from build123d import *

# Parameters (mm, degrees)
BOSS_EXTRUDE1_DEPTH = 6.35


with BuildPart() as part:
    # Sketch1 → Boss-Extrude1 (new body)
    with BuildSketch(Plane(origin=(0, 0, 0), x_dir=(1, 0, 0), z_dir=(0, 1, 0))):
        with BuildLine():
            Line((1.248119104, -4.675816263), (2.497415053, -4.675816263))
            Line((2.497415053, -4.675816263), (2.497415053, -2.923216263))
            Line((2.497415053, -2.923216263), (5.037415053, -2.923216263))
            Line((5.037415053, -2.923216263), (5.037415053, -4.675816263))
            Line((5.037415053, -4.675816263), (8.212415053, -4.675816263))
            Line((8.212415053, -4.675816263), (8.212415053, -3.02471078))
            Line((8.212415053, -3.02471078), (8.212415053, 3.32528922))
            Line((8.212415053, 3.32528922), (14.562415053, 3.32528922))
            Line((14.562415053, 3.32528922), (14.562415053, 9.67528922))
            Line((14.562415053, 9.67528922), (8.212415053, 9.67528922))
            Line((8.212415053, 9.67528922), (-101.041741874, -93.72811078))
            ThreePointArc((-101.041741874, -93.72811078), (-118.331248541, -106.150388972), (-137.459794183, -115.49591078))
            Line((-137.459794183, -115.49591078), (-137.459794183, -123.496945941))
            Line((-137.459794183, -123.496945941), (-134.284794183, -123.496945941))
            Line((-134.284794183, -123.496945941), (-134.284794183, -121.744345941))
            Line((-134.284794183, -121.744345941), (-131.744794183, -121.744345941))
            Line((-131.744794183, -121.744345941), (-131.744794183, -123.496945941))
            Line((-131.744794183, -123.496945941), (-130.474794183, -123.496945941))
            Line((-130.474794183, -123.496945941), (-130.474794183, -126.544805297))
            Line((-130.474794183, -126.544805297), (-131.744794183, -126.544805297))
            Line((-131.744794183, -126.544805297), (-131.744794183, -128.297405297))
            Line((-131.744794183, -128.297405297), (-134.284794183, -128.297405297))
            Line((-134.284794183, -128.297405297), (-134.284794183, -126.544805297))
            Line((-134.284794183, -126.544805297), (-137.459794183, -126.544805297))
            Line((-137.459794183, -126.544805297), (-137.459794183, -134.54591078))
            Line((-137.459794183, -134.54591078), (-143.809794183, -134.54591078))
            Line((-143.809794183, -134.54591078), (-143.809794183, -140.89591078))
            Line((-143.809794183, -140.89591078), (-137.459794183, -140.89591078))
            Line((-137.459794183, -140.89591078), (-28.205637256, -37.49251078))
            ThreePointArc((-28.205637256, -37.49251078), (-10.916130589, -25.070232587), (8.212415053, -15.72471078))
            Line((8.212415053, -15.72471078), (8.212415053, -7.723675619))
            Line((8.212415053, -7.723675619), (5.037415053, -7.723675619))
            Line((5.037415053, -7.723675619), (5.037415053, -9.476275619))
            Line((5.037415053, -9.476275619), (2.497415053, -9.476275619))
            Line((2.497415053, -9.476275619), (2.497415053, -7.723675619))
            Line((2.497415053, -7.723675619), (1.248119104, -7.723675619))
            Line((1.248119104, -7.723675619), (1.248119104, -4.675816263))
        make_face()
    extrude(amount=BOSS_EXTRUDE1_DEPTH)


solid = part.part
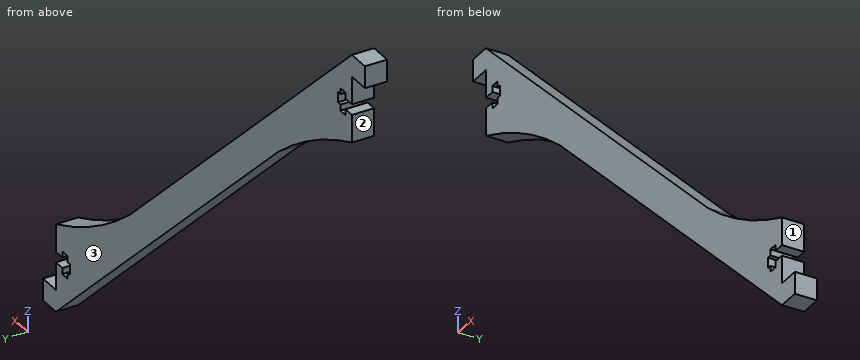
Model file for the job. Use its own axes, mm. Face numbers are marked on the shaded views. A direction names the side the tool comes from. Coordinates: 2 decimals unless noted, no trailing zeros. Write each loop counter-clockwise with the first axis right and the second up, starting at its lowest first coordinate (ties: lowest second). Pieces come first, ordered by that corner, then holes. Notation, with made-up numbers: (2.25, 11.25) - (33.25, 11.25) arc R28 ccw to (33.25, 36.25) - close; hole circle Ø3 at (12, 1.5). An arc over 180 degrees is marked (long way). Write each question's results on one line, items separated by ' | '. Start each with the question number.
1) Flat gauge pins, fed straight in: P1, Ø1, axis at y = 4.5, z = 79, coming from the +X side; P2, Ø1, axis at x = -131, y = 2, coming from the +Z side; P3, Ø2, axis at x = -133, y = 3, coming from the +Z side. Where does each tip first touch, or does it go through?
2) Cut at A-A (x = -124.5). Write the cut outline in (y, z), then the cut area to 3 significant figures.
3) Probe line 1 along X through (y, z) = (3.5, 123); line 2 along X through (y, z) = (0.5, 8.5); line 3 along X through (y, z) = (1, 5). List the from-to ranges inside material, lowest first. Write a range as from..to.
4) 3-axis set-ups, long thin cutter, end or side, ignore diameter. For the marked faces 1, 2 and 3: which of +Z, -Z, +X, -X, +Y, -Y reach the whole face in a straight line?
5) Cut at B-B (z = 23.5). Write the cut outline in (x, y).
Returned:
1) P1: x = -71.53 | P2: z = 135.26 | P3: z = 137.62
2) outline: (0, 109.61) - (6.35, 109.61) - (6.35, 128.63) - (0, 128.63) - close | area: 121 mm^2
3) line 1: -137.46..-134.28, -131.74..-118.55 | line 2: -10.99..2.5, 5.04..8.21 | line 3: -7.29..1.25
4) face 1: +Z, +X, +Y, -Y | face 2: -Z, -X, +Y, -Y | face 3: +Z, -Z, +X, -X, +Y
5) outline: (-26.84, 0) - (-8.21, 0) - (-8.21, 6.35) - (-26.84, 6.35) - close
